Input: part model. Units: mm. Frame: model coordinates. Face numbers are marked on the shaded views. A direction names the side the tool comes from. Coordinates: 2 decimals unless noted, no trailing zeros. Write each loop counter-clockwise with the first axis right and the second up, starting at its lowest first coordinate (ties: lowest second). Pieces come first, ordered by that corner, then holes. Notation, with made-up numbers: (-10, -5.5) - (39, -5.5) arc R33 ccw to (39, 22.5) - close; hole circle Ø5 at (40.25, -5.5). An arc over 180 degrees is marked (long way). Use CSV: the item, a comma, the result in double quotes.
```python
from build123d import *

# Parameters (mm, degrees)
SKETCH2_W                                  = 100
SKETCH2_H                                  = 50
BOSS_EXTRUDE1_DEPTH                        = 2
CUT_EXTRUDE1_REACH                         = 57.937
SKETCH3_R                                  = 1.5
SKETCH4_W                                  = 5
SKETCH4_H                                  = 5
BOSS_EXTRUDE2_DEPTH                        = 50
MIRROR1_AT_THE_SECOND_PLANE_COPY_1_SKETC_W = 5
MIRROR1_AT_THE_SECOND_PLANE_COPY_1_SKETC_H = 5
MIRROR1_AT_THE_SECOND_PLANE_COPY_1_DEPTH   = 50
SKETCH5_W                                  = 100
SKETCH5_H                                  = 50
BOSS_EXTRUDE3_DEPTH                        = 2


with BuildPart() as part:
    # Sketch2 → Boss-Extrude1 (new body)
    with BuildSketch(Plane(origin=(0, 0, 0), x_dir=(1, 0, 0), z_dir=(0, 1, 0))):
        Rectangle(SKETCH2_W, SKETCH2_H)
    extrude(amount=BOSS_EXTRUDE1_DEPTH)

    # Sketch3 → Cut-Extrude1 (cut, up to next)
    with BuildSketch(Plane(origin=(0, 2, 0), x_dir=(1, 0, 0), z_dir=(0, 1, 0)), mode=Mode.PRIVATE) as cut_extrude1_sk1:
        with Locations(Location((0, 0, 0), (0, 0, 270))):
            Circle(SKETCH3_R)
    cut_extrude1_tool1 = extrude(cut_extrude1_sk1.sketch, amount=-CUT_EXTRUDE1_REACH, mode=Mode.PRIVATE) & part.part
    add(cut_extrude1_tool1.solids().sort_by_distance((0, 2, 0))[0], mode=Mode.SUBTRACT)

    # Sketch4 → Boss-Extrude2 (add)
    with BuildSketch(Plane(origin=(0, 2, 0), x_dir=(1, 0, 0), z_dir=(0, 1, 0))):
        with Locations((-44.5, 19.5)):
            Rectangle(SKETCH4_W, SKETCH4_H)
    boss_extrude2 = extrude(amount=BOSS_EXTRUDE2_DEPTH)

    # Mirror1: Boss-Extrude2 across plane
    add(boss_extrude2.mirror(Plane.XY))

    # Mirror1 at the second plane: Boss-Extrude2 across plane
    add(boss_extrude2.mirror(Plane(origin=(0, 0, 0), x_dir=(0, 0, 1), z_dir=(1, 0, 0))))

    # Mirror1 at the second plane copy 1 sketc → Mirror1 at the second plane copy 1 (add)
    with BuildSketch(Plane(origin=(0, 2, 0), x_dir=(-1, 0, 0), z_dir=(0, 1, 0))):
        with Locations((-44.5, 19.5)):
            Rectangle(MIRROR1_AT_THE_SECOND_PLANE_COPY_1_SKETC_W, MIRROR1_AT_THE_SECOND_PLANE_COPY_1_SKETC_H)
    extrude(amount=MIRROR1_AT_THE_SECOND_PLANE_COPY_1_DEPTH)

    # Sketch5 → Boss-Extrude3 (add)
    with BuildSketch(Plane(origin=(0, 52, 0), x_dir=(1, 0, 0), z_dir=(0, 1, 0))):
        Rectangle(SKETCH5_W, SKETCH5_H)
    extrude(amount=BOSS_EXTRUDE3_DEPTH)


solid = part.part
```
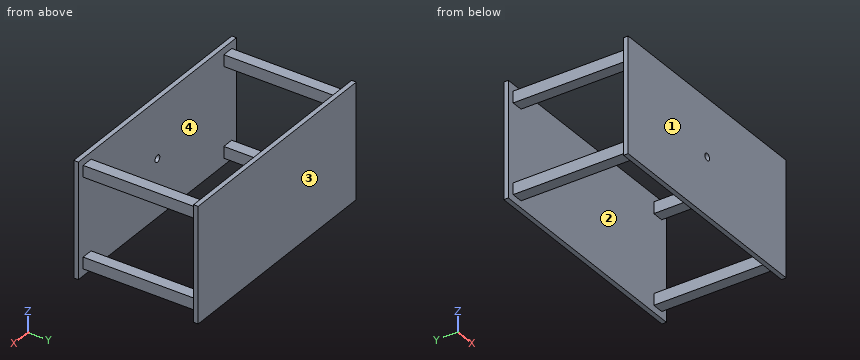
(1) Cut plane A-A on z = -11.5. Return loops of the section in (x, y).
Check values:
outline,"(-50, 0) - (50, 0) - (50, 2) - (-50, 2) - close; (-50, 52) - (50, 52) - (50, 54) - (-50, 54) - close"
(2) Pin query (flat end, axial travel): pin 1 Ø2.5 at (x, y) = (-44, 27) entering from -Z; pin 2 Ø1.5 at (x, y) = (43.5, 16.5) entering from +Z; pin 3 Ø4 at (y, z) = (29, -18.5) entering from -X. Return the tip coordinate at first contact, or that it passes through.
Check values:
pin 1,"z = -22"
pin 2,"z = 22"
pin 3,"x = -47"
(3) Reachability of the marked faces 1 and 2 from +Z, -Z, +X, -X, +Y, -Y: full face, straight path, thin tool, end or side. Return the list, or none.
Check values:
face 1,"+Z, -Z, +X, -X, -Y"
face 2,"none"
(4) Cut plane B-B on x = 0. Return loops of the section in (y, z), and give its area (3 significant figures).
Check values:
outline,"(0, -25) - (2, -25) - (2, -1.5) - (0, -1.5) - close; (0, 1.5) - (2, 1.5) - (2, 25) - (0, 25) - close; (52, -25) - (54, -25) - (54, 25) - (52, 25) - close"
area,"194 mm^2"
(5) Cut plane C-C on z = 0. Return loops of the section in (x, y).
Check values:
outline,"(-50, 0) - (-1.5, 0) - (-1.5, 2) - (-50, 2) - close; (-50, 52) - (50, 52) - (50, 54) - (-50, 54) - close; (1.5, 0) - (50, 0) - (50, 2) - (1.5, 2) - close"
(6) Ray query, probe 1 along X at (y, z) = (26.5, -21); probe 2 along Y at (x, z) = (-38.5, -12.5); probe 3 along X at (y, z) = (1, 0). Return the intervals inside material, ascending. Write a range as from..to.
Check values:
probe 1,"-47..-42, 42..47"
probe 2,"0..2, 52..54"
probe 3,"-50..-1.5, 1.5..50"
(7) Cut plane D-D on y = 18. Return loops of the section in (x, z), and give its area (3 significant figures).
Check values:
outline,"(-47, -22) - (-42, -22) - (-42, -17) - (-47, -17) - close; (-47, 17) - (-42, 17) - (-42, 22) - (-47, 22) - close; (42, -22) - (47, -22) - (47, -17) - (42, -17) - close; (42, 17) - (47, 17) - (47, 22) - (42, 22) - close"
area,"100 mm^2"
(8) Draft query along X for the marked faces 3 and 4. Return one class per face: pulls with the +X half, pulls with the -X half, needs draft (parallel to the pull), parting line crosses it, or undercut.
Check values:
face 3,"needs draft"
face 4,"undercut"
